Can you work these out from the model? Positions are in its coordinate system, mm. A direction names the side the tool comes from. Give positions to 0.01 mm unless a question says otherwise; leave off trailing zeros. Order: outer loops, then holes, each group sorted by start corner. A loop starts at its lowest first (then second) coordinate and runs counter-clockwise, first axis right, second up. Notation, with made-up numbers: M -22.5,-40 L 0.5,-40 A20 ccw 0.5,-15 Z; hole C 50,21.25 d3. An arc over 180 degrees is marked long. Answer as a JSON object with one key per item and string values.
```python
from build123d import *

# Parameters (mm, degrees)
SKETCH1_R           = 9.55
SKETCH1_R_2         = 2
BOSS_EXTRUDE1_DEPTH = 3


with BuildPart() as part:
    # Sketch1 → Boss-Extrude1 (new body)
    with BuildSketch(Plane.XY):
        Circle(SKETCH1_R)
        with BuildLine():
            Line((-1.25, 0.829156198), (1.25, 0.829156198))
            ThreePointArc((1.25, 0.829156198), (0, -1.5), (-1.25, 0.829156198))
        make_face(mode=Mode.SUBTRACT)
        with Locations((0, -5)):
            Circle(SKETCH1_R_2, mode=Mode.SUBTRACT)
        with Locations((-4.330127019, 2.5)):
            Circle(SKETCH1_R_2, mode=Mode.SUBTRACT)
        with Locations((4.330127019, 2.5)):
            Circle(SKETCH1_R_2, mode=Mode.SUBTRACT)
    extrude(amount=BOSS_EXTRUDE1_DEPTH)


solid = part.part
```
1) I want a section at C-C on x = 3. Write out the boundary of the cut face in (y, z).
Results found:
{"outline": "M -9.07,0 L 1.01,0 L 1.01,3 L -9.07,3 Z; M 3.99,0 L 9.07,0 L 9.07,3 L 3.99,3 Z"}
2) I want a section at A-A on x = 0. Write out the boundary of the cut face in (y, z), and give its area (3 significant figures).
Results found:
{"outline": "M -9.55,0 L -7,0 L -7,3 L -9.55,3 Z; M -3,0 L -1.5,0 L -1.5,3 L -3,3 Z; M 0.83,0 L 9.55,0 L 9.55,3 L 0.83,3 Z", "area": "38.3 mm²"}
3) I want a section at D-D on z = 2. Write out the boundary of the cut face in (x, y).
Results found:
{"outline": "C 0,0 d19.1; hole C -4.33,2.5 d4; hole C 0,-5 d4; hole M -1.25,0.83 A1.5 ccw long 1.25,0.83 Z; hole C 4.33,2.5 d4"}
4) I'm going to push flat-ended pins straight in: pin 1 Ø3.5 at (x, y) = (4.33, 2.5) entering from +Z; pin 2 Ø1 at (x, z) = (5.5, 1) entering from -Y. Where does each tip first touch, or does it pass through?
Results found:
{"pin 1": "passes through", "pin 2": "stops at y = -8.14"}
5) Thinking about a two-plate mould opening in X: for faces 3 (the face through (0, -1.5, 1.5)), 4 (the face through (0, -2, 3)), 5 (the face through (-7.58, -5.81, 1.48)), which applies, pulls with the +X half, pulls with the -X half, needs draft (parallel to the pull), parting line crosses it, or undercut?
Results found:
{"face 3": "undercut", "face 4": "needs draft", "face 5": "parting line crosses it"}
6) I need wall thicknesses on L1, parallel to Y at x = 0, z = 1.1; L2, parallel to Y at x = 0.5, z = 1.9; L3, parallel to Y at x = -3.25, z = 0.5. Which ranges of each line are inside material? Lowest first, please.
Results found:
{"L1": "y = -9.55 to -7, -3 to -1.5, 0.83 to 9.55", "L2": "y = -9.54 to -6.94, -3.06 to -1.41, 0.83 to 9.54", "L3": "y = -8.98 to 0.82, 4.18 to 8.98"}
7) For faces 1 (the face through (0, 0.829, 1)), 2 (the face through (0, -2, 0)), which set-ups out of +Z, -Z, +X, -X, +Y, -Y let a thin tool reach every point of the face, with its end or its side?
Results found:
{"face 1": "+Z, -Z", "face 2": "-Z, +X, -X, +Y, -Y"}
8) I want a section at B-B on y = 0. Write out the boundary of the cut face in (x, z), and give its area (3 significant figures).
Results found:
{"outline": "M -9.55,0 L -1.5,0 L -1.5,3 L -9.55,3 Z; M 1.5,0 L 9.55,0 L 9.55,3 L 1.5,3 Z", "area": "48.3 mm²"}
